Read the model definition and answer for the solid it produces. Units are mm, in the model's axes. A direction names the side the tool comes from. Coordinates: 2 decimals unless noted, no trailing zeros.
from build123d import *

# Parameters (mm, degrees)
F1_DEPTH = 3.175
F4_D     = 1.016
F5_SIZE  = 0.1524


with BuildPart() as f1:
    # F0 (on Top) → F1 (new body)
    with BuildSketch(Plane.XY):
        with BuildLine():
            ThreePointArc((5.2705, -0.4572), (4.526551, -2.253251), (2.7305, -2.9972))
            Line((2.7305, -2.9972), (1.0795, -2.9972))
            Line((1.0795, -2.9972), (-1.0795, -2.9972))
            Line((-1.0795, -2.9972), (-2.7305, -2.9972))
            ThreePointArc((-2.7305, -2.9972), (-6.322602, -4.485098), (-7.8105, -8.0772))
            Line((-7.8105, -8.0772), (-7.8105, -8.9916))
            ThreePointArc((-7.8105, -8.9916), (-6.322602, -12.583702), (-2.7305, -14.0716))
            Line((-2.7305, -14.0716), (-1.0795, -14.0716))
            Line((-1.0795, -14.0716), (1.0795, -14.0716))
            Line((1.0795, -14.0716), (2.7305, -14.0716))
            ThreePointArc((2.7305, -14.0716), (4.526551, -14.815549), (5.2705, -16.6116))
            Line((5.2705, -16.6116), (5.2705, -17.526))
            ThreePointArc((5.2705, -17.526), (4.526551, -19.322051), (2.7305, -20.066))
            Line((2.7305, -20.066), (1.0795, -20.066))
            Line((1.0795, -20.066), (-1.0795, -20.066))
            Line((-1.0795, -20.066), (-6.35, -20.066))
            Line((-6.35, -20.066), (-6.35, -22.606))
            Line((-6.35, -22.606), (2.7305, -22.606))
            ThreePointArc((2.7305, -22.606), (6.322602, -21.118102), (7.8105, -17.526))
            Line((7.8105, -17.526), (7.8105, -16.6116))
            ThreePointArc((7.8105, -16.6116), (6.685893, -13.423925), (3.81, -11.647622))
            ThreePointArc((3.81, -11.647622), (3.273358, -11.560689), (2.7305, -11.5316))
            Line((2.7305, -11.5316), (1.0795, -11.5316))
            Line((1.0795, -11.5316), (-1.0795, -11.5316))
            Line((-1.0795, -11.5316), (-2.7305, -11.5316))
            ThreePointArc((-2.7305, -11.5316), (-4.526551, -10.787651), (-5.2705, -8.9916))
            Line((-5.2705, -8.9916), (-5.2705, -8.0772))
            ThreePointArc((-5.2705, -8.0772), (-4.526551, -6.281149), (-2.7305, -5.5372))
            Line((-2.7305, -5.5372), (-1.0795, -5.5372))
            Line((-1.0795, -5.5372), (1.0795, -5.5372))
            Line((1.0795, -5.5372), (2.7305, -5.5372))
            ThreePointArc((2.7305, -5.5372), (6.322602, -4.049302), (7.8105, -0.4572))
            Line((7.8105, -0.4572), (7.8105, 0.4572))
            ThreePointArc((7.8105, 0.4572), (6.322602, 4.049302), (2.7305, 5.5372))
            Line((2.7305, 5.5372), (-6.35, 5.5372))
            Line((-6.35, 5.5372), (-6.35, 2.9972))
            Line((-6.35, 2.9972), (-1.0795, 2.9972))
            Line((-1.0795, 2.9972), (1.0795, 2.9972))
            Line((1.0795, 2.9972), (2.7305, 2.9972))
            ThreePointArc((2.7305, 2.9972), (4.526551, 2.253251), (5.2705, 0.4572))
            Line((5.2705, 0.4572), (5.2705, -0.4572))
        make_face()
    extrude(amount=F1_DEPTH)

    # F4 (through all)
    with Locations(Plane.XZ.offset(22.606)):
        with Locations((0, 1.5875)):
            Hole(F4_D / 2)

    # F5
    f5_edges = [f1.edges().sort_by_distance(p)[0] for p in [
        (4.526551, 2.253251, 3.175),
        (5.2705, 0, 3.175),
        (4.526551, -2.253251, 3.175),
        (0, -2.9972, 3.175),
        (-6.322602, -4.485098, 3.175),
        (-7.8105, -8.5344, 3.175),
        (-6.322602, -12.583702, 3.175),
        (0, -14.0716, 3.175),
        (4.526551, -14.815549, 3.175),
        (5.2705, -17.0688, 3.175),
        (4.526551, -19.322051, 3.175),
        (-1.80975, -20.066, 3.175),
        (-6.35, -21.336, 3.175),
        (-1.80975, -22.606, 3.175),
        (6.322602, -21.118102, 3.175),
        (7.8105, -17.0688, 3.175),
        (6.322602, -13.019498, 3.175),
        (0, -11.5316, 3.175),
        (-4.526551, -10.787651, 3.175),
        (-5.2705, -8.5344, 3.175),
        (-4.526551, -6.281149, 3.175),
        (0, -5.5372, 3.175),
        (6.322602, -4.049302, 3.175),
        (7.8105, 0, 3.175),
        (6.322602, 4.049302, 3.175),
        (-1.80975, 5.5372, 3.175),
        (-6.35, 4.2672, 3.175),
        (-1.80975, 2.9972, 3.175),
        (4.526551, 2.253251, 0),
        (5.2705, 0, 0),
        (4.526551, -2.253251, 0),
        (0, -2.9972, 0),
        (-6.322602, -4.485098, 0),
        (-7.8105, -8.5344, 0),
        (-6.322602, -12.583702, 0),
        (0, -14.0716, 0),
        (4.526551, -14.815549, 0),
        (5.2705, -17.0688, 0),
        (4.526551, -19.322051, 0),
        (-1.80975, -20.066, 0),
        (-6.35, -21.336, 0),
        (-1.80975, -22.606, 0),
        (6.322602, -21.118102, 0),
        (7.8105, -17.0688, 0),
        (6.322602, -13.019498, 0),
        (0, -11.5316, 0),
        (-4.526551, -10.787651, 0),
        (-5.2705, -8.5344, 0),
        (-4.526551, -6.281149, 0),
        (0, -5.5372, 0),
        (6.322602, -4.049302, 0),
        (7.8105, 0, 0),
        (6.322602, 4.049302, 0),
        (-1.80975, 5.5372, 0),
        (-6.35, 4.2672, 0),
        (-1.80975, 2.9972, 0),
    ]]
    chamfer(f5_edges, length=F5_SIZE)


solid = f1.part
Q1. Straight lines are drawn through the part: probe 1 along Y at (x, z) = (-2.5, 1.3); probe 2 along Y at (x, z) = (4.25, 2.9); probe 3 along Y at (x, z) = (-6, 0.6). For each, find the intervals that lie inside material, in ascending order.
Findings below:
probe 1: y = -22.61 to -20.07, -14.07 to -11.53, -5.54 to -3, 3 to 5.54
probe 2: y = -22.37 to -19.56, -14.58 to -11.76, -5.3 to -2.49, 2.49 to 5.3
probe 3: y = -22.61 to -20.07, -12.88 to -4.19, 3 to 5.54
Q2. Which of the six approach directions +Z, -Z, +X, -X, +Y, -Y give full straight-line access (tool end or side, diameter ignored) to faces 5 (the face through (7.81, 0, 2)), 6 (the face through (4.55, -2.23, 1.57)), 7 (the face through (-4.507, -10.807, 1.567))?
Findings below:
face 5: +Z, -Z, +X, +Y, -Y
face 6: +Z, -Z, -X
face 7: +Z, -Z, +X
Q3. A cutting plane is placed at A-A (x = -2.25). Count the separate pieces of the cut face and the enclosed holes in it, then the cut area to 3 significant figures.
Findings below:
separate pieces: 4
enclosed holes: 0
area: 32.1 mm2
Q4. Flat-ended cylindrical pins translate along their axes: pin 1 Ø0.7 at (y, z) = (-17, 1.5) entering from -X; pin 2 Ø0.8 at (y, z) = (4.5, 2) entering from -X; pin 3 Ø0.7 at (y, z) = (-8.5, 1) entering from +X. Find the tip coordinate at first contact, or state that the pin passes through.
Findings below:
pin 1: stops at x = 5.27
pin 2: stops at x = -6.35
pin 3: stops at x = -5.27
Q5. Determine the mould class of faces 1 (the face through (-1, -5.537, 2)), 2 (the face through (-5.27, -8.5, 1.6)), 3 (the face through (-2, 5.537, 2)), 4 (the face through (2, -5, 3.175)) for opening direction Y: +Y half, -Y half, draft (parallel to the pull), parting line (faces both ways), or undercut.
Findings below:
face 1: undercut
face 2: undercut
face 3: +Y half
face 4: draft
